from build123d import *

# Parameters (mm, degrees)
SKETCH1_W           = 104.1
SKETCH1_H           = 132.64
SKETCH1_W_2         = 96.1
SKETCH1_H_2         = 124.64
BOSS_EXTRUDE1_DEPTH = 11
SKETCH3_R           = 3.025
CUT_EXTRUDE1_DEPTH  = 124.919943512
LPATTERN1_COUNT     = 4
LPATTERN1_PITCH     = 29
BOSS_EXTRUDE2_DEPTH = 2.1


with BuildPart() as part:
    # Sketch1 → Boss-Extrude1 (new body)
    with BuildSketch(Plane(origin=(0, 0, 0), x_dir=(1, 0, 0), z_dir=(0, 1, 0))):
        Rectangle(SKETCH1_W, SKETCH1_H)
        Rectangle(SKETCH1_W_2, SKETCH1_H_2, mode=Mode.SUBTRACT)
    extrude(amount=BOSS_EXTRUDE1_DEPTH)

    # Sketch3 → Cut-Extrude1 (cut, through all)
    with BuildSketch(Plane(origin=(52.05, 0, 0), x_dir=(0, 0, -1), z_dir=(1, 0, 0))):
        with Locations((-49.82, 6.5)):
            Circle(SKETCH3_R)
    cut_extrude1 = extrude(amount=-CUT_EXTRUDE1_DEPTH, mode=Mode.SUBTRACT)

    # LPattern1: Cut-Extrude1 ×4
    with Locations(*[(0, 0, -i * LPATTERN1_PITCH) for i in range(1, LPATTERN1_COUNT)]):
        add(cut_extrude1, mode=Mode.SUBTRACT)

    # Sketch5 → Boss-Extrude2 (add)
    with BuildSketch(Plane.XZ):
        Polygon((48.05, 62.32), (48.05, 26.32), (52.05, 26.32), (52.05, 66.32), (-52.05, 66.32), (-52.05, 26.32), (-48.05, 26.32), (-48.05, 62.32), align=None)
        Polygon((-48.05, -22.26), (-52.05, -22.26), (-52.05, -66.32), (52.05, -66.32), (52.05, -22.26), (48.05, -22.26), (48.05, -62.32), (-48.05, -62.32), align=None)
    extrude(amount=BOSS_EXTRUDE2_DEPTH)


solid = part.part
Verification items for the finished model (mm, model axes). A direction names the side the tool comes from. Coordinates: 2 decimals unless noted, no trailing zeros. Order: outer loops, then holes, each group sorted by start corner. A loop starts at its lowest first (then second) coordinate and runs counter-clockwise, first axis right, second up.
Item 1: Section check B-B, the plane z = -13.5. Enter the section's corners in (x, y), then the cut area to 3 significant figures.
Filled in:
outline: (-52.05, 0) - (-48.05, 0) - (-48.05, 11) - (-52.05, 11) - close; (48.05, 0) - (52.05, 0) - (52.05, 11) - (48.05, 11) - close
area: 88.0 mm2
Item 2: Section check D-D, the plane y = 6.5. Give the number of separate pieces and of enclosed holes in the cut face, then the cut area to 3 significant figures.
Filled in:
separate pieces: 8
enclosed holes: 0
area: 1,640 mm2
Item 3: Section check A-A, the plane z = 49.82. Enter the section's corners in (x, y) (3 decimals).
Filled in:
outline: (-52.05, -2.1) - (-48.05, -2.1) - (-48.05, 3.475) - (-52.05, 3.475) - close; (-52.05, 9.525) - (-48.05, 9.525) - (-48.05, 11) - (-52.05, 11) - close; (48.05, -2.1) - (52.05, -2.1) - (52.05, 3.475) - (48.05, 3.475) - close; (48.05, 9.525) - (52.05, 9.525) - (52.05, 11) - (48.05, 11) - close
Item 4: Material ranges on L1, parallel to Z at x = -34, y = 8; L2, parallel to X at y = 1, z = -39; L3, parallel to Y at x = -49.55, z = 20.82 (3 decimals), recorded low to high.
Filled in:
L1: z = -66.32 to -62.32, 62.32 to 66.32
L2: x = -52.05 to -48.05, 48.05 to 52.05
L3: y = 0 to 3.475, 9.525 to 11
Item 5: Section check C-C, the plane x = -7. Enter the section's corners in (y, z).
Filled in:
outline: (-2.1, -66.32) - (11, -66.32) - (11, -62.32) - (-2.1, -62.32) - close; (-2.1, 62.32) - (11, 62.32) - (11, 66.32) - (-2.1, 66.32) - close
Item 6: Depth check by flat-ended pin: pin 1 (1.5 mm diameter, centred on y = 7.5, z = -5.5, fed in from +X); pin 2 (3 mm diameter, centred on x = -50, z = -1, fed in from -Y). Enter the tip coordinate at first touch or a pass-through.
Filled in:
pin 1: stops at x = 52.05
pin 2: stops at y = 0
Item 7: Release check for a two-part mould opening along Z. For faces 4 (the face through (50.078, 3.547, 50.476)), 5 (the face through (-1, 4, -66.32)), 6 (the face through (-50.02, 4.66, -34.78)), 7 (the face through (52.05, 5, -1)) record: +Z half, -Z half, draft (parallel to the pull), parting line (faces both ways), or undercut.
Filled in:
face 4: undercut
face 5: -Z half
face 6: undercut
face 7: draft
Item 8: Access from +Z, -Z, +X, -X, +Y, -Y to the whole of each face (thin tool, end or side, straight path). Record for faces 1 (the face through (-50.022, 5.341, 18.026)), 2 (the face through (48.05, 5, 1)), 3 (the face through (50, 0, 2)).
Filled in:
face 1: +X, -X
face 2: +Y, -Y
face 3: +X, -X, -Y
